Autodesk Fusion 360 part; units mm, degrees
sketch "Esquisse1" plane through (0, 0, 0) normal (0, 0, 1) x (1, 0, 0)
  line L0 (0, 0) -> (-36, 0)
  line L1 (-36, 0) -> (-36, 80)
  line L2 (-36, 80) -> (0, 80)
  line L3 (0, 80) -> (0, 0)
  line L4 (-36.5, 80.5) -> (0.5, 80.5)
  line L5 (0.5, 80.5) -> (0.5, -0.5)
  line L6 (0.5, -0.5) -> (-36.5, -0.5)
  line L7 (-36.5, -0.5) -> (-36.5, 80.5)
  line L8 (-38.5, 82.5) -> (2.5, 82.5)
  line L9 (2.5, 82.5) -> (2.5, -2.5)
  line L10 (2.5, -2.5) -> (-38.5, -2.5)
  line L11 (-38.5, -2.5) -> (-38.5, 82.5)
  circle A0 centre (4, 70.04) radius 1.5
  circle A1 centre (4, 70.04) radius 3
  circle A2 centre (-40, 19.95) radius 1.5
  circle A3 centre (-40, 19.95) radius 3
  line L12 (-42.5, 85.5) -> (6.5, 85.5)
  line L13 (6.5, 85.5) -> (6.5, -5.5)
  line L14 (6.5, -5.5) -> (-42.5, -5.5)
  line L15 (-42.5, -5.5) -> (-42.5, 85.5)
  dimension "d1" = 36
  dimension "d2" = 80
  dimension "d3" = 0.5
  dimension "d4" = 0.5
  dimension "d5" = 0.5
  dimension "d6" = 0.5
  dimension "d7" = 2
  dimension "d8" = 2
  dimension "d9" = 2
  dimension "d10" = 2
  dimension "d11" = 3
  dimension "d12" = 9.96
  dimension "d13" = 4
  dimension "d14" = 6
  dimension "d15" = 3
  dimension "d16" = 4
  dimension "d17" = 6
  dimension "d18" = 19.95
  dimension "d19" = 3
  dimension "d20" = 4
  dimension "d21" = 4
  dimension "d22" = 3
extrude "Extrusion1" add sketch "Esquisse1" along normal blind 3 contours L8 L9 L11 A1 A3 L12 L13 L15 | L8 L9 L10 L11 A1 A3 | L11 A3 | L11 A3 L15 | L9 A1 L13 | L9 A1 | L9 L10 L11 A1 A3 L13 L14 L15
sketch "Esquisse2" plane through (0, 0, 3) normal (0, 0, 1) x (-1, 0, 0)
  circle A0 centre (40, -19.95) radius 1.5
  circle A1 centre (-4, -70.04) radius 1.5
  line L0 (-0.5, 0.5) -> (36.5, 0.5)
  line L1 (36.5, 0.5) -> (36.5, -80.5)
  line L2 (36.5, -80.5) -> (-0.5, -80.5)
  line L3 (-0.5, -80.5) -> (-0.5, 0.5)
  line L4 (42.5, 5.5) -> (-6.5, 5.5)
  line L5 (-6.5, 5.5) -> (-6.5, -85.5)
  line L6 (-6.5, -85.5) -> (42.5, -85.5)
  line L7 (42.5, -85.5) -> (42.5, 5.5)
  line L8 (36.5, -80.5) -> (33.5, -80.5)
  line L9 (33.5, -80.5) -> (33.5, 0.5)
  line L10 (33.5, 0.5) -> (36.5, 0.5)
  line L11 (36.5, 0.5) -> (36.5, -80.5)
  line L12 (-0.5, -80.5) -> (2.5, -80.5)
  line L13 (2.5, -80.5) -> (2.5, 0.5)
  line L14 (2.5, 0.5) -> (-0.5, 0.5)
  line L15 (-0.5, 0.5) -> (-0.5, -80.5)
  dimension "d25" = 3
  dimension "d26" = 3
extrude "Extrusion2" add sketch "Esquisse2" along normal blind 2 contours L0 L2 L3 L12 L13 L14 L15 | L0 L1 L2 L8 L9 L10 L11 | L4 L5 L6 L7
Model file for the job. Use its own axes, mm. A direction names the side the tool comes from. Give positions to 0.01 mm unless a question says otherwise; leave off trailing zeros. Loops run counter-clockwise (first coordinate to the right, second up) from the corner with the lowest first, then second, coordinate; pieces in that order, holes last.
Item 1: Which spindle directions (+Z, -Z, +X, -X, +Y, -Y) get a long thin tool onto all of the face, cutting with end or side? Do faces 5 (the face through (-38, 44, 0)), 6 (the face through (-33.5, 41, 4)), 7 (the face through (0.5, 41, 1)). Say none if no direction does.
Check values:
face 5: -Z, +X, -X, +Y, -Y
face 6: +Z, -Z
face 7: -Z
Item 2: Slice it at C-C (x = -8). Write the cut outline in (y, z), plus the area to 3 significant figures.
Check values:
outline: (-5.5, 0) - (-0.5, 0) - (-0.5, 5) - (-5.5, 5) - close; (80.5, 0) - (85.5, 0) - (85.5, 5) - (80.5, 5) - close
area: 50.0 mm2
Item 3: Drill centre lines: line 1 along X through (y, z) = (19.95, 3.9); line 2 along X through (y, z) = (70, 2.4); line 3 along X through (y, z) = (65, 3.2). Where is each one in solid material? Low to high.
Check values:
line 1: x = -42.5 to -41.5, -38.5 to -33.5, -2.5 to 6.5
line 2: x = -42.5 to -36.5, 0.5 to 2.5, 5.5 to 6.5
line 3: x = -42.5 to -33.5, -2.5 to 6.5
Item 4: Drop a flat-ended pin along its axis: P1, Ø2, axis at x = -3, y = 35, coming from the -Z side. Give the stop position or say it passes through.
Check values:
P1: stops at z = 3
Item 5: Mould opens along X. For faces 1 (the face through (-42.5, 39, 2)), 2 (the face through (-18, 85.5, 2)), 3 (the face through (-40.099, 21.447, 3.021)), 4 (the face through (-1, 39, 3)) say: +X half, -X half, draft (parallel to the pull), parting line (faces both ways), or undercut.
Check values:
face 1: -X half
face 2: draft
face 3: undercut
face 4: undercut
Item 6: Slice it at B-B (y = 35.5). Write the cut outline in (x, z), plus the area to 3 significant figures.
Check values:
outline: (-42.5, 0) - (-36.5, 0) - (-36.5, 3) - (-33.5, 3) - (-33.5, 5) - (-42.5, 5) - close; (-2.5, 3) - (0.5, 3) - (0.5, 0) - (6.5, 0) - (6.5, 5) - (-2.5, 5) - close
area: 72.0 mm2
Item 7: Slice it at A-A (z = 1.7). Write the cut outline in (x, y), plus the area to 3 significant figures.
Check values:
outline: (-42.5, -5.5) - (6.5, -5.5) - (6.5, 85.5) - (-42.5, 85.5) - close; hole circle Ø3 at (-40, 19.95); hole (-36.5, -0.5) - (0.5, -0.5) - (0.5, 80.5) - (-36.5, 80.5) - close; hole circle Ø3 at (4, 70.04)
area: 1,450 mm2
